Could you check a few things on this model? Use its own coordinates, in mm. A direction names the side the tool comes from. Give positions to 0.01 mm unless a question says otherwise; leave off trailing zeros. Loops run counter-clockwise (first coordinate to the right, second up) from the corner with the lowest first, then second, coordinate; pieces in that order, holes last. Notation, with made-up numbers: (-4.75, -23) - (31.25, -23) arc R22 cw to (31.25, -13) - close; hole circle Ø5 at (89, 24). An arc over 180 degrees is marked (long way). Write each question's results on one line, items separated by ' | '. Start each with the question number.
1) I'm going to push flat-ended pins straight in: pin 1 (4 mm diameter, centred on x = 7, y = -15, fed in from +Z); pin 2 (17 mm diameter, centred on x = 31.5, z = 20.5, fed in from +Y); pin 3 (3 mm diameter, centred on x = 25.5, z = 24.5, fed in from -Y). Where does each tip first touch, or does it pass through?
2) On a 3-axis mill with a long thin cutter (end or side, diameter ignored), from which of +Z, -Z, +X, -X, +Y, -Y can I reach the whole of each face in a straight line? I mean faces 1 (the face through (43.14, -14.8, 19.65)), 2 (the face through (6, -15, 9)), 3 (the face through (18, -24, 19)), 4 (the face through (37, -11.247, 17)). Say none if no direction works.
3) I want a section at D-D, the plane y = -1.5. Write out the boundary of the cut face in (x, z), and give its area (3 significant figures).
4) I want a section at B-B, the plane x = 55. Write out the boundary of the cut face in (y, z).
5) If I drill on probe 1 along Z at (x, y) = (51.5, -24); probe 2 along Y at (x, z) = (44, 13.5); probe 3 along X at (y, z) = (-15.5, 11), over which ranges is the centre line in solid material (lowest first)? Write a range as [from, to].
6) If we mould it in two halves opening along X, with no side actions, what happens to faces 5 (the face through (43, -24, 9)), 6 (the face through (5.993, -11.305, 19.647)), 7 (the face through (69, -15, 4))? For each: +X half, -X half, draft (parallel to the pull), parting line (faces both ways), or undercut.
7) I want a section at A-A, the plane z = 4. Write out the boundary of the cut face in (x, y), and give its area (3 significant figures).
8) I want a section at C-C, the plane z = 15. Write out the boundary of the cut face in (x, y).
from build123d import *

# Parameters (mm, degrees)
F1_DEPTH = 9
F3_DEPTH = 21
F4_W     = 51
F4_H     = 7
F5_DEPTH = 21
F7_DEPTH = 25
F8_R     = 3.75
F9_DEPTH = 21


with BuildPart() as f1:
    # F0 (on Top) → F1 (new body)
    with BuildSketch(Plane.XY):
        with BuildLine():
            ThreePointArc((0, 0), (-4.019238, -15), (0, -30))
            Line((0, -30), (60, -30))
            Line((60, -30), (69, -21))
            Line((69, -21), (69, -9))
            Line((69, -9), (60, 0))
            Line((60, 0), (0, 0))
        make_face()
    extrude(amount=F1_DEPTH)

    # F2 (on face) → F3 (join)
    with BuildSketch(Plane.XY.offset(9)):
        with BuildLine():
            Line((0, -30), (18, -30))
            Line((18, -30), (18, 0))
            Line((18, 0), (0, 0))
            ThreePointArc((0, 0), (-4.019238, -15), (0, -30))
        make_face()
    extrude(amount=F3_DEPTH)

    # F4 (on face) → F5 (join)
    with BuildSketch(Plane.XY.offset(9)):
        with Locations((43.5, -14.746526)):
            Rectangle(F4_W, F4_H)
    extrude(amount=F5_DEPTH)

    # F6 (on face) → F7 (cut)
    with BuildSketch(Plane.XZ.offset(18.246526)):
        Polygon((69, 30), (18, 30), (69, 9), align=None)
    extrude(amount=-F7_DEPTH, mode=Mode.SUBTRACT)

    # F8 (on face) → F9 (cut)
    with BuildSketch(Plane.XY.offset(30)):
        with Locations((6.480922, -15.023556)):
            Circle(F8_R)
    extrude(amount=-F9_DEPTH, mode=Mode.SUBTRACT)


solid = f1.part
Answers:
1) pin 1: stops at z = 9 | pin 2: stops at y = -11.25 | pin 3: stops at y = -18.25
2) face 1: +Z, +X, +Y, -Y | face 2: +Z | face 3: +Z, +X, -Y | face 4: +Z, +X, +Y
3) outline: (-0.81, 0) - (61.5, 0) - (61.5, 9) - (18, 9) - (18, 30) - (-0.81, 30) - close | area: 956 mm2
4) outline: (-30, 0) - (0, 0) - (0, 9) - (-11.25, 9) - (-11.25, 14.76) - (-18.25, 14.76) - (-18.25, 9) - (-30, 9) - close
5) probe 1: z = [0, 9] | probe 2: y = [-18.25, -11.25] | probe 3: x = [-4.02, 2.76], [10.2, 64.14]
6) face 5: draft | face 6: undercut | face 7: +X half
7) outline: (0, -30) - (60, -30) - (69, -21) - (69, -9) - (60, 0) - (0, 0) arc R30 ccw to start | area: 2,070 mm2
8) outline: (0, -30) - (18, -30) - (18, -18.25) - (54.43, -18.25) - (54.43, -11.25) - (18, -11.25) - (18, 0) - (0, 0) arc R30 ccw to start; hole circle Ø7.5 at (6.48, -15.02)
